from build123d import *

# Parameters (mm, degrees)
SKETCH1_W           = 25.4
SKETCH1_H           = 40.4
BOSS_EXTRUDE1_DEPTH = 10
SKETCH2_W           = 25.4
SKETCH2_H           = 25.4
BOSS_EXTRUDE2_DEPTH = 50.54
SKETCH3_R           = 1.2303
CUT_EXTRUDE1_DEPTH  = 20
SKETCH4_R           = 2.9
CUT_EXTRUDE2_DEPTH  = 66.937406682
FILLET1_R           = 3
FILLET2_R           = 12.7


with BuildPart() as part:
    # Sketch1 → Boss-Extrude1 (new body)
    with BuildSketch(Plane(origin=(0, 0, 0), x_dir=(1, 0, 0), z_dir=(0, 1, 0))):
        with Locations((0, 20.2)):
            Rectangle(SKETCH1_W, SKETCH1_H)
    extrude(amount=BOSS_EXTRUDE1_DEPTH)

    # Sketch2 → Boss-Extrude2 (add)
    with BuildSketch(Plane(origin=(0, 10, 0), x_dir=(1, 0, 0), z_dir=(0, 1, 0))):
        with Locations((0, 27.7)):
            Rectangle(SKETCH2_W, SKETCH2_H)
    extrude(amount=BOSS_EXTRUDE2_DEPTH)

    # Sketch3 → Cut-Extrude1 (cut)
    with BuildSketch(Plane(origin=(0, 60.54, 0), x_dir=(1, 0, 0), z_dir=(0, 1, 0))):
        with Locations(Location((-6.35, 34.05, 0), (0, 0, 270))):
            Circle(SKETCH3_R)
        with Locations(Location((6.35, 21.35, 0), (0, 0, 270))):
            Circle(SKETCH3_R)
    extrude(amount=-CUT_EXTRUDE1_DEPTH, mode=Mode.SUBTRACT)

    # Sketch4 → Cut-Extrude2 (cut, through all)
    with BuildSketch(Plane(origin=(0, 10, 0), x_dir=(1, 0, 0), z_dir=(0, 1, 0))):
        with Locations(Location((0, 7.5, 0), (0, 0, 270))):
            Circle(SKETCH4_R)
    extrude(amount=-CUT_EXTRUDE2_DEPTH, mode=Mode.SUBTRACT)

    # Fillet1
    fillet1_edges = [part.edges().sort_by_distance(p)[0] for p in [
        (12.7, 10, -7.5),
        (-12.7, 10, -7.5),
        (-12.7, 35.27, -15),
        (12.7, 35.27, -15),
        (0, 10, 0),
        (-12.7, 30.27, -40.4),
        (12.7, 30.27, -40.4),
    ]]
    fillet(fillet1_edges, radius=FILLET1_R)

    # Fillet2
    # the kernel refuses this fillet: 12.7 mm, written as the material it takes off along each edge
    with BuildSketch(Plane(origin=(0, 10, -12.7), x_dir=(-1, 0, 0), z_dir=(0, 0, -1))) as fillet2_piece_1:
        with BuildLine():
            CenterArc((9.7, -3), 3, 0, 90)
            Line((12.7, -3), (12.7, 0))
            Line((12.7, 0), (9.7, 0))
        make_face()
    revolve(axis=Axis((0, 10, -12.7), (0, 1, 0)), revolution_arc=90, mode=Mode.SUBTRACT)
    with BuildSketch(Plane(origin=(0, 10, -12.7), x_dir=(0, 0, 1), z_dir=(-1, 0, 0))) as fillet2_piece_2:
        with BuildLine():
            CenterArc((9.7, -3), 3, 0, 90)
            Line((12.7, -3), (12.7, 0))
            Line((12.7, 0), (9.7, 0))
        make_face()
    revolve(axis=Axis((0, 10, -12.7), (0, 1, 0)), revolution_arc=90, mode=Mode.SUBTRACT)
    with BuildSketch(Plane(origin=(12.7, -31.75, 0), x_dir=(0, 0, -1), z_dir=(0, 1, 0))) as fillet2_piece_3:
        with BuildLine():
            CenterArc((FILLET2_R, FILLET2_R), FILLET2_R, 180, 90)
            Line((0, FILLET2_R), (0, 0))
            Line((0, 0), (FILLET2_R, 0))
        make_face()
    extrude(amount=41.75, mode=Mode.SUBTRACT)
    with BuildSketch(Plane(origin=(-12.7, -31.75, 0), x_dir=(0, 0, -1), z_dir=(0, 1, 0))) as fillet2_piece_4:
        with BuildLine():
            CenterArc((FILLET2_R, -FILLET2_R), FILLET2_R, 90, 90)
            Line((0, -FILLET2_R), (0, 0))
            Line((0, 0), (FILLET2_R, 0))
        make_face()
    extrude(amount=41.75, mode=Mode.SUBTRACT)


solid = part.part
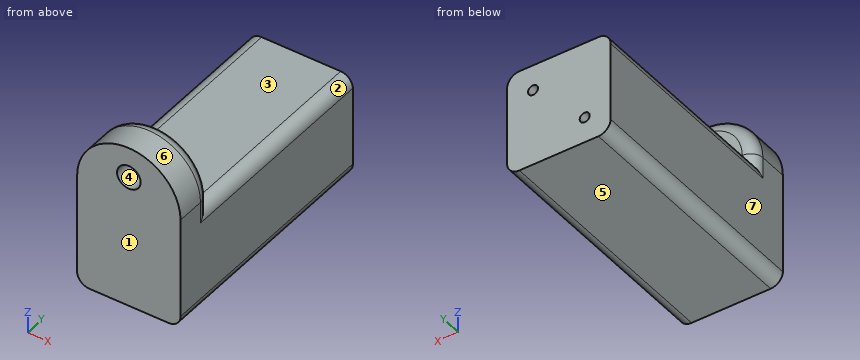
Read the model definition and answer for the solid it produces. Units are mm, in the model's axes. Face numbers are marked on the shaded views. A direction names the side the tool comes from. Coordinates: 2 decimals unless noted, no trailing zeros. Loops run counter-clockwise (first coordinate to the right, second up) from the corner with the lowest first, then second, coordinate; pieces in that order, holes last. Notation, with made-up numbers: (9.25, 89.25) -> (38.25, 89.25) arc R10 cw to (38.25, 102.25) -> close; hole circle Ø1 at (78.25, 74). An arc over 180 degrees is marked (long way). Write item = value, one per line. Start each with the question number.
1) The mould has two halves that part along Z. Classify the marked faces 4, 5, 6 and 7: pulls with the +Z half, pulls with the -Z half, needs draft (parallel to the pull), parting line crosses it, or undercut.
2) Find the intervals of material crossed by L1, parallel to X at y = 55.5, z = -21.35; L2, parallel to X at y = 48, z = -34; L3, parallel to Y at x = 3.25, z = -14, in increasing order. Write a range as from..to.
3) The part is cut by section D-D, the plane z = -14. Determine the outline of the cut face in (x, y), plus the area to 3 significant figures.
4) The part is cut by section A-A, the plane x = 0. Determine the outline of the cut face in (y, z).
5) The part is cut by section B-B, the plane z = -21.35. Determine the outline of the cut face in (x, y).
6) For the marked faces 1, 2 and 3, determine the directions among +Z, -Z, +X, -X, +Y, -Y from which every point of the face is accessible in a straight line to the end or side of a thin tool.
7) The part is cut by section C-C, the plane y = 18. Determine the outline of the cut face in (x, z), plus the area to 3 significant figures.
8) Given P1, Ø12, axis at x = -6.5, y = 18.5, coming from the +Z side; P2, Ø3.5, axis at x = 4, z = -6, coming from the +Y side; P3, Ø2, axis at x = -6.35, z = -34.05, coming from the -Y side; P4, Ø1.2, axis at x = 6, z = -21, coming from the +Y side, each flat-ended and moving along its own axis, determine where each tip first touches the part or whether it passes through.
Result:
q1.face_4 = undercut
q1.face_5 = pulls with the -Z half
q1.face_6 = pulls with the +Z half
q1.face_7 = needs draft
q2.L1 = -12.7..5.12, 7.58..12.7
q2.L2 = -12.7..-7.58, -5.12..12.7
q2.L3 = 0..10
q3.outline = (-12.7, 0) -> (12.7, 0) -> (12.7, 7) arc R3 ccw to (9.7, 10) -> (-9.7, 10) arc R3 ccw to (-12.7, 7) -> close
q3.area = 250 mm²
q4.outline = (0, -40.4) -> (60.54, -40.4) -> (60.54, -15) -> (10, -15) -> (10, -10.4) -> (0, -10.4) -> close; (0, -4.6) -> (10, -4.6) -> (10, -3) arc R3 ccw to (7, 0) -> (0, 0) -> close
q5.outline = (-12.7, 0) -> (12.7, 0) -> (12.7, 60.54) -> (7.58, 60.54) -> (7.58, 40.54) -> (5.12, 40.54) -> (5.12, 60.54) -> (-12.7, 60.54) -> close
q6.face_1 = +Z, -Z, +X, -X, -Y
q6.face_2 = +Z, +X, +Y
q6.face_3 = +Z, +X, -X, +Y
q7.outline = (-12.7, -37.4) arc R3 ccw to (-9.7, -40.4) -> (9.7, -40.4) arc R3 ccw to (12.7, -37.4) -> (12.7, -18) arc R3 ccw to (9.7, -15) -> (-9.7, -15) arc R3 ccw to (-12.7, -18) -> close
q7.area = 637 mm²
q8.P1 = -15
q8.P2 = 10
q8.P3 = 0
q8.P4 = 40.54
